Source: CAD feature listing. Evaluate the final solid. Frame: model axes, mm. Give positions to 0.01 mm unless a question says otherwise; leave off trailing zeros. Order: outer loops, then holes, each group sorted by start corner. A loop starts at its lowest first (then second) coordinate and runs counter-clockwise, first axis right, second up.
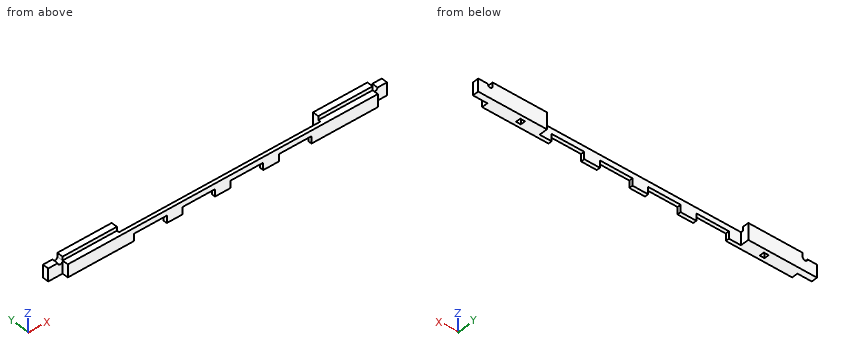
```python
from build123d import *

# Parameters (mm, degrees)
F1_DEPTH = 5
F0_W     = 128.6
F0_H     = 1.6
F2_DEPTH = 2.5
F3_W     = 2
F3_H     = 2
F4_DEPTH = 2
F5_W     = 2
F5_H     = 2
F6_DEPTH = 2
F8_DEPTH = 3.5


with BuildPart() as f1:
    # F0 (on Front) → F1 (new body)
    with BuildSketch(Plane.XZ):
        Polygon((64.3, 0.177778), (64.3, 5.477778), (-64.3, 5.477778), (-64.3, 0.177778), (-36.75, 0.177778), (-36.75, 3.177778), (-23.25, 3.177778), (-23.25, 0.177778), (-16.75, 0.177778), (-16.75, 3.177778), (-3.25, 3.177778), (-3.25, 0.177778), (3.25, 0.177778), (3.25, 3.177778), (16.75, 3.177778), (16.75, 0.177778), (23.25, 0.177778), (23.25, 3.177778), (36.75, 3.177778), (36.75, 0.177778), align=None)
    extrude(amount=F1_DEPTH)

    # F0 (on Front) → F2 (join)
    with BuildSketch(Plane.XZ):
        with BuildLine():
            Line((-64.3, 0.177778), (-64.3, 5.477778))
            ThreePointArc((-64.3, 5.477778), (-65.3, 4.477778), (-66.3, 5.477778))
            Line((-66.3, 5.477778), (-70.25, 5.477778))
            Line((-70.25, 5.477778), (-70.25, 0.177778))
            Line((-70.25, 0.177778), (-64.3, 0.177778))
        make_face()
        with Locations((0, 6.277778)):
            Rectangle(F0_W, F0_H)
        with BuildLine():
            ThreePointArc((66.3, 5.477778), (65.3, 4.477778), (64.3, 5.477778))
            Line((64.3, 5.477778), (64.3, 0.177778))
            Line((64.3, 0.177778), (70.25, 0.177778))
            Line((70.25, 0.177778), (70.25, 5.477778))
            Line((70.25, 5.477778), (66.3, 5.477778))
        make_face()
    extrude(amount=F2_DEPTH)

    # F3 (on face) → F4 (cut)
    with BuildSketch(Plane(origin=(0, 0, 0.177778), x_dir=(1, 0, 0), z_dir=(0, 0, -1))):
        with Locations((50.525, 2.5)):
            Rectangle(F3_W, F3_H)
    extrude(amount=-F4_DEPTH, mode=Mode.SUBTRACT)

    # F5 (on face) → F6 (cut)
    with BuildSketch(Plane(origin=(0, 0, 0.177778), x_dir=(1, 0, 0), z_dir=(0, 0, -1))):
        with Locations((-50.525, 2.5)):
            Rectangle(F5_W, F5_H)
    extrude(amount=-F6_DEPTH, mode=Mode.SUBTRACT)

    # F7 (on face) → F8 (cut)
    with BuildSketch(Plane(origin=(0, 0, 0), x_dir=(-1, 0, 0), z_dir=(0, 1, 0))):
        Polygon((-41.75, 7.077778), (-41.75, 0.177778), (-36.75, 0.177778), (-36.75, 3.177778), (-23.25, 3.177778), (-23.25, 0.177778), (-16.75, 0.177778), (-16.75, 3.177778), (-3.25, 3.177778), (-3.25, 0.177778), (3.25, 0.177778), (3.25, 3.177778), (16.75, 3.177778), (16.75, 0.177778), (23.25, 0.177778), (23.25, 3.177778), (36.75, 3.177778), (36.75, 0.177778), (41.75, 0.177778), (41.75, 7.077778), align=None)
    extrude(amount=-F8_DEPTH, mode=Mode.SUBTRACT)


solid = f1.part
```
1) Material intervals for L1, parallel to X at y = -1.35, z = 5.25; L2, parallel to X at y = -2.3, z = 6.25; L3, parallel to X at y = -2.85, z = 1.5 (3 decimals), sorted ascending.
Report:
L1: x = -70.25 to -66.27, -64.33 to -41.75, 41.75 to 64.33, 66.27 to 70.25
L2: x = -64.3 to -41.75, 41.75 to 64.3
L3: x = -64.3 to -51.525, -49.525 to -41.75, 41.75 to 49.525, 51.525 to 64.3
2) Section query A-A, the plane y = -0.75. Return the cut outline in (x, z).
Report:
outline: (-70.25, 0.18) - (-41.75, 0.18) - (-41.75, 7.08) - (-64.3, 7.08) - (-64.3, 5.48) arc R1 cw to (-66.3, 5.48) - (-70.25, 5.48) - close; (41.75, 0.18) - (70.25, 0.18) - (70.25, 5.48) - (66.3, 5.48) arc R1 cw to (64.3, 5.48) - (64.3, 7.08) - (41.75, 7.08) - close
3) Section query B-B, the plane x = 44.5. Return the cut outline in (y, z), and give its area (3 significant figures).
Report:
outline: (-5, 0.18) - (0, 0.18) - (0, 7.08) - (-2.5, 7.08) - (-2.5, 5.48) - (-5, 5.48) - close
area: 30.5 mm2
4) Section query D-D, the plane x = 21.5. Return the cut outline in (y, z).
Report:
outline: (-5, 0.18) - (-3.5, 0.18) - (-3.5, 5.48) - (-5, 5.48) - close
5) Section query C-C, the plane x = -32. Return the cut outline in (y, z).
Report:
outline: (-5, 3.18) - (-3.5, 3.18) - (-3.5, 5.48) - (-5, 5.48) - close
6) Pin query (flat end, axial travel): pin 1 (1.6 mm diameter, centred on x = 9.5, y = -4.5, fed in from -Z); pin 2 (4 mm diameter, centred on x = -31.5, z = 4.5, fed in from +Y); pin 3 (1.6 mm diameter, centred on y = -4.5, z = 1, fed in from -X). Return the tip coordinate at first contact, or that it passes through.
Report:
pin 1: stops at z = 3.18
pin 2: stops at y = -3.5
pin 3: stops at x = -64.3
